```python
from build123d import *

# Parameters (mm, degrees)
F0_R     = 3.175
F1_DEPTH = 25.4


with BuildPart() as f1:
    # F0 (on Front) → F1 (new body, symmetric)
    with BuildSketch(Plane.XZ):
        with BuildLine():
            ThreePointArc((-98.135353981, 38.3118497444), (-82.4605407052, 49.3130634455), (-67.60536263, 37.2279420774))
            Line((-67.60536263, 37.2279420774), (-70.8167565395, 69.7700589479))
            Line((-70.8167565395, 69.7700589479), (-73.4987966791, 96.9480589479))
            ThreePointArc((-73.4987966791, 96.9480589479), (-83.0237966791, 87.4230589479), (-92.5487966791, 96.9480589479))
            Line((-92.5487966791, 96.9480589479), (-98.135353981, 38.3118497444))
        make_face()
        with Locations((-88.1071984768, 69.7700589479)):
            Circle(F0_R, mode=Mode.SUBTRACT)
        with BuildLine():
            ThreePointArc((-98.8394449745, 32.0766020597), (-82.6839530039, 17.5766969624), (-67.1639389713, 32.7548501134))
            Line((-67.1639389713, 32.7548501134), (-67.2323477549, 33.4480589479))
            Line((-67.2323477549, 33.4480589479), (-79.8487966791, 33.4480589479))
            ThreePointArc((-79.8487966791, 33.4480589479), (-83.0237966791, 30.2730589479), (-86.1987966791, 33.4480589479))
            Line((-86.1987966791, 33.4480589479), (-98.8987966791, 33.4480589479))
            Line((-98.8987966791, 33.4480589479), (-98.8394449745, 32.0766020597))
        make_face()
        with BuildLine():
            Line((-79.8487966791, 33.4480589479), (-67.2323477549, 33.4480589479))
            Line((-67.2323477549, 33.4480589479), (-67.60536263, 37.2279420774))
            ThreePointArc((-67.60536263, 37.2279420774), (-82.4605407052, 49.3130634455), (-98.135353981, 38.3118497444))
            ThreePointArc((-98.135353981, 38.3118497444), (-98.7067746675, 35.9097304159), (-98.8987966791, 33.4480589479))
            Line((-98.8987966791, 33.4480589479), (-86.1987966791, 33.4480589479))
            ThreePointArc((-86.1987966791, 33.4480589479), (-83.0237966791, 36.6230589479), (-79.8487966791, 33.4480589479))
        make_face()
        with BuildLine():
            ThreePointArc((-83.0237966791, -16.9372670215), (-81.5065627429, -17.025326906), (-80.0097040665, -17.2883239844))
            Line((-80.0097040665, -17.2883239844), (-69.4052307289, -18.5234466834))
            Line((-69.4052307289, -18.5234466834), (-67.1639389713, 32.7548501134))
            ThreePointArc((-67.1639389713, 32.7548501134), (-82.6839530039, 17.5766969624), (-98.8394449745, 32.0766020597))
            Line((-98.8394449745, 32.0766020597), (-96.1507458476, -30.0519410521))
            Line((-96.1507458476, -30.0519410521), (-96.1384707097, -30.0519410521))
            ThreePointArc((-96.1384707097, -30.0519410521), (-92.2972716192, -20.778466112), (-83.0237966791, -16.9372670215))
        make_face()
        with BuildLine():
            ThreePointArc((-73.4987966791, 96.9480589479), (-83.0237966791, 106.4730589479), (-92.5487966791, 96.9480589479))
            ThreePointArc((-92.5487966791, 96.9480589479), (-83.0237966791, 87.4230589479), (-73.4987966791, 96.9480589479))
        make_face()
        with BuildLine():
            ThreePointArc((-79.8487966791, 96.9480589479), (-83.0237966791, 93.7730589479), (-86.1987966791, 96.9480589479))
            ThreePointArc((-86.1987966791, 96.9480589479), (-83.0237966791, 100.1230589479), (-79.8487966791, 96.9480589479))
        make_face(mode=Mode.SUBTRACT)
        with BuildLine():
            ThreePointArc((-79.9704602907, -42.80622707), (-72.7272393329, -38.1744764779), (-69.9091226485, -30.0519410521))
            ThreePointArc((-69.9091226485, -30.0519410521), (-72.7397430756, -21.9135802584), (-80.0097040665, -17.2883239844))
            Line((-80.0097040665, -17.2883239844), (-83.0237966791, -16.9372670215))
            ThreePointArc((-83.0237966791, -16.9372670215), (-92.2972716192, -20.778466112), (-96.1384707097, -30.0519410521))
            ThreePointArc((-96.1384707097, -30.0519410521), (-92.1669135373, -39.4539668469), (-82.6576798276, -43.1615037214))
            Line((-82.6576798276, -43.1615037214), (-80.3456263931, -42.8902461913))
            ThreePointArc((-80.3456263931, -42.8902461913), (-80.1577354458, -42.8496114626), (-79.9704602907, -42.80622707))
        make_face()
        with BuildLine():
            ThreePointArc((-79.8487966791, -30.0519410521), (-83.0237966791, -33.2269410521), (-86.1987966791, -30.0519410521))
            ThreePointArc((-86.1987966791, -30.0519410521), (-83.0237966791, -26.8769410521), (-79.8487966791, -30.0519410521))
        make_face(mode=Mode.SUBTRACT)
        with BuildLine():
            Line((-69.4052307289, -18.5234466834), (-69.9091226485, -30.0519410521))
            ThreePointArc((-69.9091226485, -30.0519410521), (-72.7272393329, -38.1744764779), (-79.9704602907, -42.80622707))
            Line((-79.9704602907, -42.80622707), (-38.5737966791, -37.9894410521))
            ThreePointArc((-38.5737966791, -37.9894410521), (-46.5112966791, -30.0519410521), (-38.5737966791, -22.1144410521))
            Line((-38.5737966791, -22.1144410521), (-69.4052307289, -18.5234466834))
        make_face()
        with BuildLine():
            ThreePointArc((-38.5737966791, -22.1144410521), (-46.5112966791, -30.0519410521), (-38.5737966791, -37.9894410521))
            ThreePointArc((-38.5737966791, -37.9894410521), (-32.9611366035, -35.6646011277), (-30.6362966791, -30.0519410521))
            ThreePointArc((-30.6362966791, -30.0519410521), (-32.9611366035, -24.4392809764), (-38.5737966791, -22.1144410521))
        make_face()
        with Locations((-38.5737966791, -30.0519410521)):
            Circle(F0_R, mode=Mode.SUBTRACT)
        with BuildLine():
            ThreePointArc((-80.0097040665, -17.2883239844), (-72.7397430756, -21.9135802584), (-69.9091226485, -30.0519410521))
            Line((-69.9091226485, -30.0519410521), (-69.4052307289, -18.5234466834))
            Line((-69.4052307289, -18.5234466834), (-80.0097040665, -17.2883239844))
        make_face()
    extrude(amount=F1_DEPTH, both=True)


solid = f1.part
```
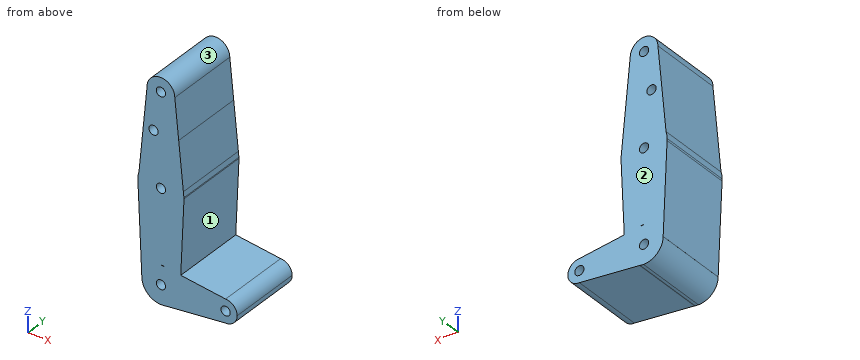
Here's how the part is built. I have some questions about the finished solid (model axes, mm). Face numbers are marked on the shaded views. Round coordinates to 2 decimals unless told otherwise and drop trailing zeros. Order: outer loops, then holes, each group sorted by start corner. A loop starts at its lowest first (then second) coordinate and runs counter-clockwise, first axis right, second up. Notation, with made-up numbers: M -31,15 L 11,15 A23 cw 11,33 Z; hole C 41,36 d10. An arc over 180 degrees is marked long. Use CSV: the item, a comma, the result in double quotes.
1) I want a section at D-D (x = -53.5). List the corners of the cut face in (y, z) for me.
Taken from the geometry:
outline,"M -25.4,-39.73 L 25.4,-39.73 L 25.4,-20.38 L -25.4,-20.38 Z"
2) I'm going to push flat-ended pins straight in: P1, Ø4, axis at x = -83.02, z = 33.45, coming from the -Y side; P2, Ø1.5, axis at y = -7, z = 7, coming from the -X side; P3, Ø3, axis at y = -18, z = -1.5, coming from the +X side; P4, Ø12, axis at y = -8.5, z = 81, coming from the +X side. Where does each tip first touch, or does it pass through?
Taken from the geometry:
P1,"through"
P2,"x = -97.79"
P3,"x = -68.6"
P4,"x = -71.33"
3) I want a section at B-B (x = -88). List the corners of the cut face in (y, z) for me.
Taken from the geometry:
outline,"M -25.4,-42.19 L 25.4,-42.19 L 25.4,66.6 L -25.4,66.6 Z; M -25.4,72.94 L 25.4,72.94 L 25.4,105.07 L -25.4,105.07 Z"
4) I want a section at C-C (z = 1.5). List the corners of the cut face in (x, y) for me.
Taken from the geometry:
outline,"M -97.52,-25.4 L -68.53,-25.4 L -68.53,25.4 L -97.52,25.4 Z"
5) I need wall thicknesses on line 1 along X through (y, z) = (13.5, -30); line 2 along X through (y, z) = (-4, 97.5); line 3 along X through (y, z) = (-11.5, 71). Which ranges of each line are inside material? Lowest first, please. Write a range as [from, to].
Taken from the geometry:
line 1,"[-96.15, -86.2], [-79.85, -41.75], [-35.4, -30.64]"
line 2,"[-92.53, -86.15], [-79.9, -73.51]"
line 3,"[-95.02, -91.03], [-85.18, -70.94]"
6) I want a section at A-A (y = 15). Count the separate pieces of the cut face and the enclosed holes in it, then the cut area to 3 significant figures.
Taken from the geometry:
separate pieces,"1"
enclosed holes,"6"
area,"4,430 mm^2"
7) If we mould it in two halves opening along Z, with no side actions, what happens to the marked faces 1, 2 and 3? For each: pulls with the +Z half, pulls with the -Z half, needs draft (parallel to the pull), parting line crosses it, or undercut.
Taken from the geometry:
face 1,"undercut"
face 2,"needs draft"
face 3,"pulls with the +Z half"
